Autodesk Inventor part; units mm, degrees
ref_plane "YZ Plane" through (0, 0, 0) normal (1, 0, 0) x (0, 1, 0)
ref_plane "XZ Plane" through (0, 0, 0) normal (0, 1, 0) x (-1, 0, 0)
ref_plane "XY Plane" through (0, 0, 0) normal (0, 0, 1) x (1, 0, 0)
sketch "Sketch1" plane through (0, 0, 0) normal (0, 0, 1) x (1, 0, 0)
  arc A0 (-71.9586, -1745.1712) -> (-70, 0) centre (-11089.4751, -860.2193) ccw
  line L0 (0, 0) -> (-70, 0)
  line L1 (0, -117.9106) -> (-61.4296, -117.9106) construction
  line L2 (0, -617.9106) -> (-39.1314, -617.9106) construction
  line L3 (0, -1117.9106) -> (-39.4794, -1117.9106) construction
  line L4 (0, -1617.9106) -> (-62.4758, -1617.9106) construction
  line L5 (-71.9586, -1745.1712) -> (0, -1745.1712)
  line L6 (0, 0) -> (0, -1745.1712)
  line L7 (0, -1735.1712) -> (-10.3553, -1745.1712)
  point P0 (-20, 0)
  dimension "d33" = 50
  dimension "d58" = 500
  dimension "d59" = 500
  dimension "d60" = 500
  dimension "d141" = 1745.171
  dimension "d148" = 70
  dimension "d149" = 11053
  dimension "d150" = 71.959
  dimension "d151" = 136
  dimension "d153" = 10
extrude "Plate3" add sketch "Sketch1" along normal blind 3 contours A0 L0 L6 L7 L5
sketch "Sketch3" plane through (-3, 0, 3) normal (1, 0, 0) x (0, 1, 0)
  line L0 (-1735.1712, 0) -> (0, 0)
  line L1 (0, 0) -> (0, 20)
  line L2 (0, 20) -> (-1735.1712, 20)
  line L3 (-1735.1712, 20) -> (-1735.1712, 0)
edge flange "Flange2" height 20 angle 90 thickness 3 bend radius 5 thickness toward (1, 0, 0) relief round relief width 3 relief depth 1.5 edges at (0, -867.5856, 3) wall of the first edge with corners at (-3, -1735.1712, 3) (-3, 0, 3) (-3, 0, -17) (-3, -1735.1712, -17)
bend "Bend2"
corner "Corner2"
sketch "Sketch5" plane through (0, 0, 0) normal (0, 0, 1) x (1, 0, 0)
  line L0 (-8, -1742.8967) -> (-8, 0)
  line L1 (-70, 0) -> (-8, 0)
  arc A0 (-71.9586, -1745.1712) -> (-70, 0) centre (-11089.4751, -860.2193) ccw
  line L2 (0, 0) -> (0, -1735.1712)
  line L3 (0, -114.5) -> (-29, -114.5)
  line L4 (0, -117.5) -> (-3, -117.5) construction
  line L5 (-3, -1735.1712) -> (-3, 0)
  line L6 (-29, -114.5) -> (-29, -117.5)
  line L7 (0, -614.5) -> (-39.2067, -614.5) construction
  line L8 (0, -1114.5) -> (-39.4004, -1114.5) construction
  line L9 (0, -1614.5) -> (-62.242, -1614.5) construction
  line L10 (-10.3553, -1745.1712) -> (-71.9586, -1745.1712)
  line L11 (0, -114.5) -> (0, -134.5)
  line L12 (-3, -114.5) -> (-3, -117.5) construction
  line L13 (0, -134.5) -> (-3, -134.5)
  line L14 (-29, -114.5) -> (-61.6597, -114.5) construction
  line L15 (-29, -117.5) -> (-61.4573, -117.5) construction
  line L16 (-3, -117.5) -> (-3, -134.5)
  line L17 (-3, -117.5) -> (-29, -117.5)
  line L18 (-3, -134.5) -> (-8, -134.5)
  line L19 (-8, -1742.8967) -> (-10.3553, -1745.1712)
  point P0 (0, 0)
  point P1 (845.25, -380.4205)
  point P2 (848, -380.4205)
  point P3 (-29, -116)
  point P4 (850, -410.4205)
  point P5 (-3, -114.5)
  point P6 (-3, -134.5)
  point P7 (-8, -117.5)
  dimension "d69" = 1735.1712
  dimension "d70" = 3
  dimension "d76" = 61.6598
  dimension "d80" = 39.2067
  dimension "d102" = 62.242
  dimension "d104" = 39.4004
  dimension "d106" = 3
  dimension "d107" = 20
  dimension "d108" = 116
  dimension "d112" = 29
  dimension "d142" = 500
  dimension "d143" = 500
  dimension "d144" = 500
extrude "Extrusion2" cut sketch "Sketch5" along normal through all both and the other way through all contours L0 L17 L5 L18 | L17 L6 L3 L0 | L0 L3 L5 L17 | L5 L3 L2 L13
pattern_linear "Rectangular Pattern3" count 4 spacing 500 along (0, -1, 0) of "Extrusion2"
chamfer "Corner Chamfer1" distance 6 angle 45 3 edges at (-8, -1617.5, 1.5) (-8, -1117.5, 1.5) (-8, -117.5, 1.5)
sketch "Sketch7" plane through (0, -1614.5, -17) normal (1, 0, 0) x (0, 0, -1)
  line L0 (-17, -130.6712) -> (-20, -130.6712)
  line L1 (0, 1000) -> (0, 1480)
  line L2 (-20, -130.6712) -> (0, -130.6712)
  line L3 (0, -130.6712) -> (0, 1129.3288)
  line L4 (0, 1129.3288) -> (-20, 1129.3288)
  line L5 (-20, 1129.3288) -> (-20, -130.6712)
  line L6 (0, 1129.3288) -> (-20, 1112.5468)
  point P0 (-17, 1614.5)
  point P1 (0, 1000)
  dimension "d154" = 1260
  dimension "d157" = 40
extrude "Extrusion3" cut sketch "Sketch7" against normal through all contours L0 L5 L6 L1 L3 L2
equation "\"БОРТ_стрингер_3_высота\" = 62"
equation "\"БОРТ_стрингер_4_высота\" = 39"
equation "\"БОРТ_стрингер_5_высота\" = 39"
equation "\"БОРТ_стрингер_6_высота\" = 62"
properties part number "MSC 313 RIB HIP" material "Stainless Steel"
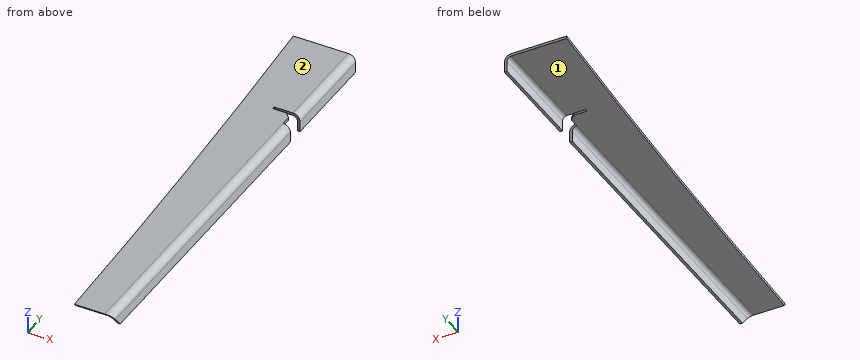
Design review of the part built by this model. Coordinates are the model's own, in mm. Face numbers are marked on the shaded views. A direction names the side the tool comes from. Round coordinates to 2 decimals unless told otherwise and drop trailing zeros. Write each loop counter-clockwise with the first axis right and the second up, starting at its lowest first coordinate (ties: lowest second). Pieces come first, ordered by that corner, then holes. Notation, with made-up numbers: (19, 13.25) -> (23, 13.25) arc R4 cw to (23, 17.25) -> close; hole circle Ø6 at (-34, -20.75). An arc over 180 degrees is marked (long way). One line per item, written item: value. Start each with the question number.
Q1. To check wall thickness, follow probe 1 along X at (y, z) = (-323, -8.75); probe 2 along Z at (x, y) = (-61.5, -114.5); probe 3 along X at (y, z) = (-480.5, -2.25). State the ranges of each line that lie inside material, in increasing order.
Q2. Add section B-B (y = -109). Give the boundary of the cut face in (x, z), then the cut area to 3 significant figures.
Q3. Insertion check: P1, Ø2.5, axis at y = -129, z = 1.5, coming from the +X side; P2, Ø2, axis at x = -8, y = -398.5, coming from the -Z side; P3, Ø2.5, axis at y = -116, z = 2, coming from the +X side. Each pin has a flat end and moves straight along its axis. Give the tip position at first contact, or say it passes through.
Q4. Add section A-A (z = -12.25). Give the boundary of the cut face in (x, y).
Q5. Tool access review of the marked faces 1 and 2: name each direction out of +Z, -Z, +X, -X, +Y, -Y from which nothing blocks a thin tool from reaching the whole face with its end or side.
Q6. Add section C-C (x = -35). Give the boundary of the cut face in (y, z), then the cut area to 3 significant figures.
Q7. Add section D-D (y = -450.5). Give the boundary of the cut face in (x, z), then the cut area to 3 significant figures.
Response:
1. probe 1: x = -3 to 0
1. probe 2: z = 0 to 3
1. probe 3: x = -3.82 to -0.49
2. outline: (-62.03, 0) -> (-8, 0) arc R5 cw to (-3, -5) -> (-3, -17) -> (0, -17) -> (0, -5) arc R8 ccw to (-8, 3) -> (-62.03, 3) -> close
2. area: 229 mm^2
3. P1: stops at x = -8
3. P2: stops at z = -0.1
3. P3: stops at x = -29
4. outline: (-3, -489.16) -> (0, -489.16) -> (0, -134.5) -> (-3, -134.5) -> close; (-3, -114.5) -> (0, -114.5) -> (0, 0) -> (-3, 0) -> close
5. face 1: -Z, -X, +Y, -Y
5. face 2: +Z, +X, -X, +Y, -Y
6. outline: (-501.95, 3) -> (-499.44, 0) -> (0, 0) -> (0, 3) -> close
6. area: 1,500 mm^2
7. outline: (-44.07, 0) -> (-8, 0) arc R5 cw to (-3, -5) -> (-3, -17) -> (0, -17) -> (0, -5) arc R8 ccw to (-8, 3) -> (-44.07, 3) -> close
7. area: 175 mm^2
